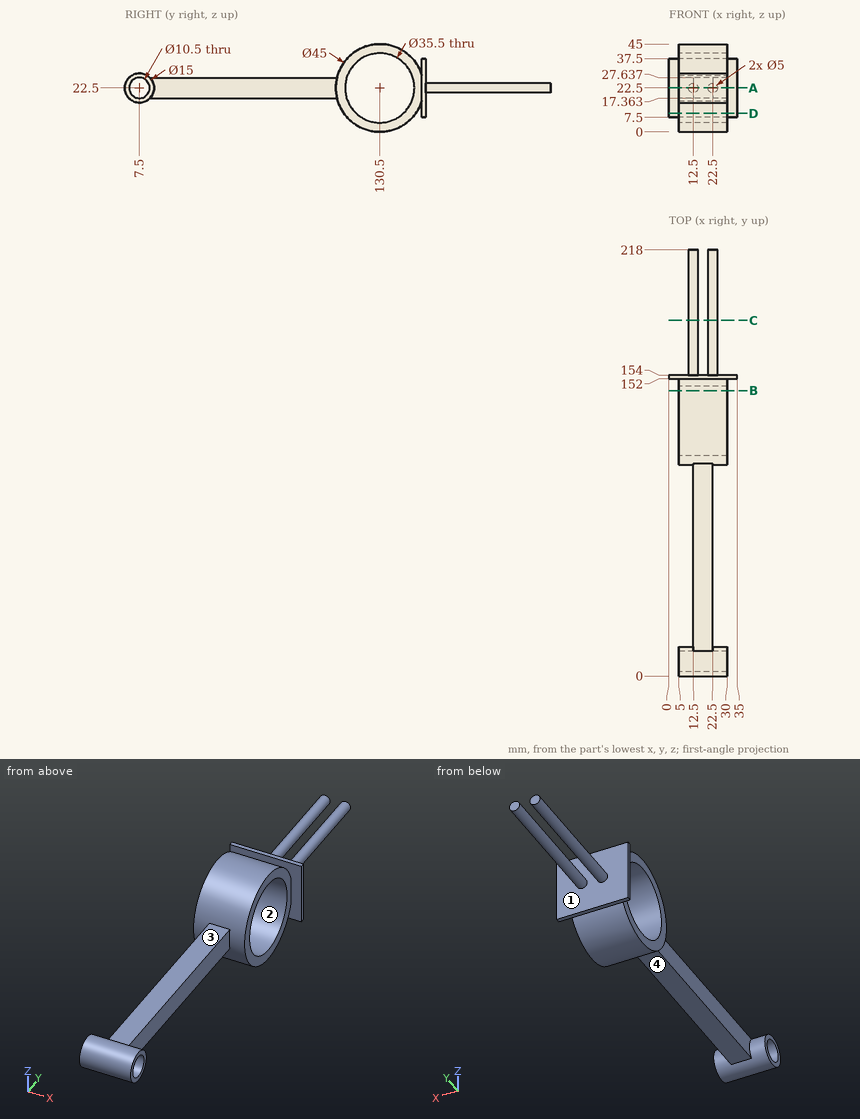
Study the drawing (mm; zero at the part's minimum x, y, z) and answer. A direction names the side the tool comes from. Coordinates: 2 decimals unless noted, no trailing zeros. Loops run counter-clockwise (first coordinate to the right, second up) from the corner with the lowest first, then second, coordinate; pieces in that order, holes last. Notation, with made-up numbers: M -18,-9 L 35,-9 A19 cw 35,18 Z; hole C 9,44.5 d8. An arc over 180 degrees is marked long. Answer as a JSON object with one key per item and string values. Group by question number.
Item 1: Section C-C (y = 182) is taken. Write down the section's boundary in (x, z).
Item 2: Section D-D (z = 9.5) is taken. Write down the section's boundary in (x, y), and give its area (3 significant figures).
Item 3: Each of these flat-tipped pins is pushed along its axis until it touches: P1, Ø13, axis at y = 139, z = 18, coming from the +X side; P2, Ø1.5, axis at x = 21, y = 145, coming from the +Z side; P3, Ø5, axis at x = 22.5, z = 9.5, coming from the -Y side; P4, Ø3, axis at x = 18, z = 32, coming from the +Y side. Where does it stop, or does it pass through?
Item 4: Determine the mould class of the marked faces 1 and 2 for opening direction Y: +Y half, -Y half, draft (parallel to the pull), parting line (faces both ways), or undercut.
Item 5: Consider L1, parallel to Z at x = 14, y = 130.5; L2, parallel to Y at x = 26.5, z = 20; L3, parallel to X at y = 18, z = 19. Determine where each line is inside the solid, lowest interval first.
Item 6: Section A-A (z = 22.5) is taken. Give the number of separate pieces and of enclosed holes in the cut face, and give its area (4 significant figures).
Item 7: Which of the six approach directions +Z, -Z, +X, -X, +Y, -Y give full straight-line access (tool end or side, diameter ignored) to the marked faces 3 and 4?
Item 8: Section B-B (y = 146) is taken. Write down the section's boundary in (x, z).
Solved:
{
 "1": {"outline": "C 12.5,22.5 d5; C 22.5,22.5 d5"},
 "2": {"outline": "M 0,152 L 35,152 L 35,154 L 0,154 Z; M 5,112.14 L 30,112.14 L 30,118.41 L 5,118.41 Z; M 5,142.59 L 30,142.59 L 30,148.86 L 5,148.86 Z", "area": "384 mm2"},
 "3": {"P1": "passes through", "P2": "stops at z = 40.31", "P3": "stops at y = 110.6", "P4": "stops at y = 154"},
 "4": {"face 1": "+Y half", "face 2": "undercut"},
 "5": {"L1": "z = 0 to 4.75, 40.25 to 45", "L2": "y = 0.43 to 2.88, 12.12 to 14.57, 108.14 to 112.93, 148.07 to 154", "L3": "x = 12.5 to 22.5"},
 "6": {"separate pieces": "3", "enclosed holes": "0", "area": "1,965 mm2"},
 "7": {"face 3": "+Z, +X, -X", "face 4": "-Z, +X, -X"},
 "8": {"outline": "M 5,6.19 L 30,6.19 L 30,13.85 L 5,13.85 Z; M 5,31.15 L 30,31.15 L 30,38.81 L 5,38.81 Z"}
}
